Design review of the part shown in the three views and the two pictorial views. Dimensions are in mm from the part's minimum x, y and z. Coordinates: 2 decimals unless noted, no trailing zeros. Loops run counter-clockwise (first coordinate to the right, second up) from the corner with the lowest first, then second, coordinate; pieces in that order, holes last. Notation, with made-up numbers: M 27,46.25 L 33,46.25 A21 ccw 33,79.25 Z; hole C -37,-11.5 d3. An arc over 180 degrees is marked long. Use CSV: the item, a comma, the result in double quotes. Start each with the question number.
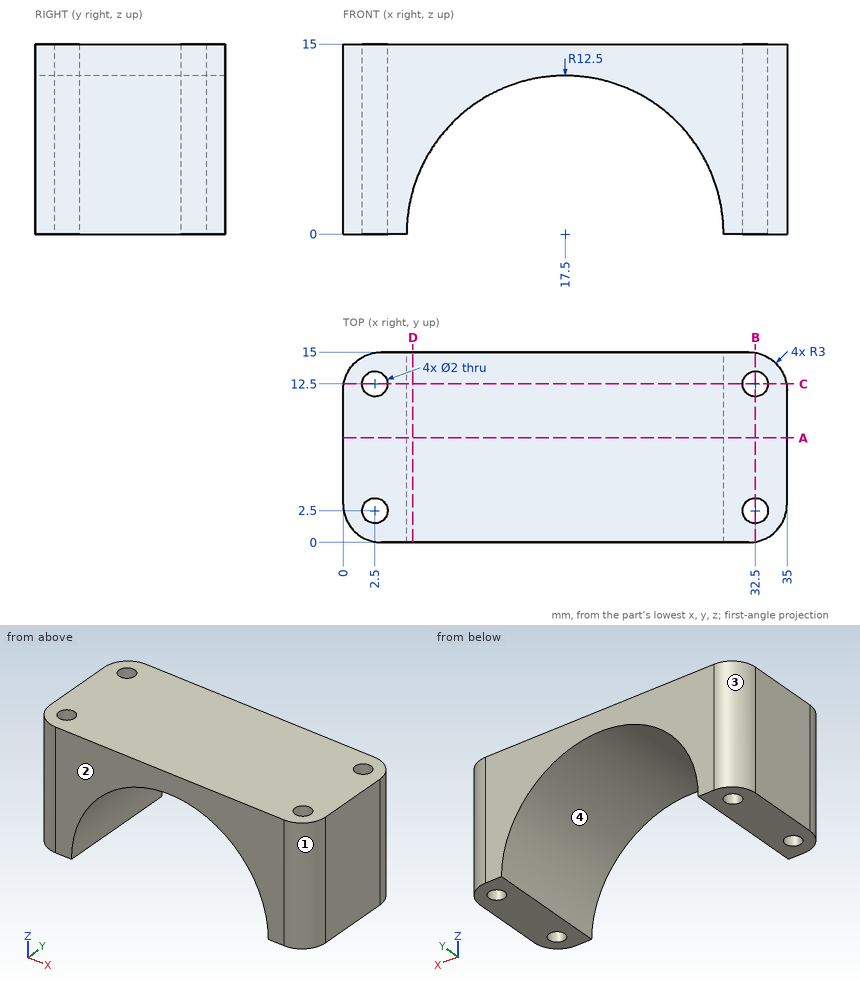
1. Add section A-A (y = 8.25). Write out the cut boundary in (x, z), plus the area to 3 significant figures.
2. Insertion check: pin 1 Ø3 at (x, z) = (8, 6.5) entering from +Y; pin 2 Ø1 at (y, z) = (13, 12) entering from -X. Each pin has a flat end and moves straight along its axis. Give the tip position at first contact, or say it passes through.
3. Draft analysis for pull direction X (two halves, no side actions). For the marked faces 1, 2, 3 and 4, state which applies: released by +X, released by -X, zero draft, split by the parting line, or undercut.
4. Add section C-C (y = 12.5). Write out the cut boundary in (x, z).
5. Add section B-B (x = 32.5). Write out the cut boundary in (y, z).
6. Add section D-D (x = 5.5). Write out the cut boundary in (y, z), plus the area to 4 significant figures.
7. To check wall thickness, follow line 1 along Y through (x, z) = (32.5, 6.75); line 2 along X through (y, z) = (7.5, 2.5); line 3 along X through (y, z) = (8, 8.75). State the ranges of each line that lie inside material, in increasing order.
Solved:
1,outline,"M 0,0 L 5,0 A12.5 cw 30,0 L 35,0 L 35,15 L 0,15 Z"
1,area,"280 mm^2"
2,pin 1,"stops at y = 15"
2,pin 2,"stops at x = 0.04"
3,face 1,"released by +X"
3,face 2,"zero draft"
3,face 3,"released by -X"
3,face 4,"undercut"
4,outline,"M 0.04,0 L 1.5,0 L 1.5,15 L 0.04,15 Z; M 3.5,0 L 5,0 A12.5 cw 30,0 L 31.5,0 L 31.5,15 L 3.5,15 Z; M 33.5,0 L 34.96,0 L 34.96,15 L 33.5,15 Z"
5,outline,"M 0.04,0 L 1.5,0 L 1.5,15 L 0.04,15 Z; M 3.5,0 L 11.5,0 L 11.5,15 L 3.5,15 Z; M 13.5,0 L 14.96,0 L 14.96,15 L 13.5,15 Z"
6,outline,"M 0,3.5 L 15,3.5 L 15,15 L 0,15 Z"
6,area,"172.5 mm^2"
7,line 1,"y = 0.04 to 1.5, 3.5 to 11.5, 13.5 to 14.96"
7,line 2,"x = 0 to 5.25, 29.75 to 35"
7,line 3,"x = 0 to 8.57, 26.43 to 35"
